Verification items for the finished model (mm, model axes). Round coordinates to 2 decimals unless told otherwise and drop trailing zeros. Order: outer loops, then holes, each group sorted by start corner. A loop starts at its lowest first (then second) coordinate and runs counter-clockwise, first axis right, second up. Notation, with made-up numbers: M 54,67.25 L 107,67.25 A23 ccw 107,81.25 Z; hole C -5.75,18 d3. An arc over 180 degrees is marked long. Answer as a JSON object with one key per item and string values. Group by question number.
```python
from build123d import *

# Parameters (mm, degrees)
SKETCH1_W           = 228.6
SKETCH1_H           = 101.6
BOSS_EXTRUDE1_DEPTH = 12.7
SKETCH2_R           = 7.9375
CUT_EXTRUDE1_DEPTH  = 12.7


with BuildPart() as part:
    # Sketch1 → Boss-Extrude1 (new body)
    with BuildSketch(Plane(origin=(0, 0, 0), x_dir=(0, 0, -1), z_dir=(1, 0, 0))):
        Rectangle(SKETCH1_W, SKETCH1_H)
    extrude(amount=-BOSS_EXTRUDE1_DEPTH)

    # Sketch2 → Cut-Extrude1 (cut)
    with BuildSketch(Plane(origin=(0, 0, 0), x_dir=(0, 0, -1), z_dir=(1, 0, 0))):
        with Locations((-95.1865, 5.2705)):
            Circle(SKETCH2_R)
    cut_extrude1 = extrude(amount=-CUT_EXTRUDE1_DEPTH, mode=Mode.SUBTRACT)

    # Mirror1: Cut-Extrude1 across plane
    add(cut_extrude1.mirror(Plane.XY), mode=Mode.SUBTRACT)


solid = part.part
```
Q1. Release check for a two-part mould opening along Z. For faces 1 (the face through (-6, -1, -114.3)), 2 (the face through (-6.261, 7.655, 87.616)), 3 (the face through (-6.261, 7.655, -87.616)), 4 (the face through (-12.7, 1, 2)) record: released by +Z, released by -Z, zero draft, split by the parting line, or undercut.
Q2. Thickness scan on line 1 (Z direction, x = -10.25, y = -2). Record the ranges inside material, lowest first. Write a range as from..to.
Q3. Cross-section at A-A, the plane x = -7.5. Record the cut outline in (y, z) (1 decimal), then the cut area to 3 significant figures.
Conclusion:
{
 "1": {"face 1": "released by -Z", "face 2": "undercut", "face 3": "undercut", "face 4": "zero draft"},
 "2": {"line 1": "-114.3..-98.37, -92..92, 98.37..114.3"},
 "3": {"outline": "M -50.8,-114.3 L 50.8,-114.3 L 50.8,114.3 L -50.8,114.3 Z; hole C 5.3,-95.2 d15.9; hole C 5.3,95.2 d15.9", "area": "22,800 mm2"}
}
